Geometry: final body of the model. Coordinates: model frame, mm. A direction names the side the tool comes from. Give positions to 0.01 mm unless a question says otherwise; leave off trailing zeros. Write each loop counter-clockwise with the first axis right and the second up, starting at its lowest first coordinate (ties: lowest second). Pieces come first, ordered by that corner, then holes.
Autodesk Inventor part; units mm, degrees
ref_plane "YZ Plane" through (0, 0, 0) normal (1, 0, 0) x (0, 1, 0)
ref_plane "XZ Plane" through (0, 0, 0) normal (0, 1, 0) x (-1, 0, 0)
ref_plane "XY Plane" through (0, 0, 0) normal (0, 0, 1) x (1, 0, 0)
sketch "Sketch1" plane through (0, 0, 0) normal (0, 1, 0) x (-1, 0, 0)
  line L0 (0, 0) -> (25.4, 0)
  line L1 (25.4, 0) -> (25.4, -19.05)
  line L2 (25.4, -19.05) -> (0, -19.05)
  line L3 (0, -19.05) -> (0, 0)
  line L4 (25.4, -9.525) -> (38.1, -9.525)
  line L5 (38.1, -9.525) -> (34.3696, 9.525)
  line L6 (34.3696, 9.525) -> (0, 0)
  line L7 (38.1, -9.525) -> (34.3696, -28.575)
  line L8 (34.3696, -28.575) -> (0, -19.05)
  line L9 (-0.8514, -15.5194) -> (31.9128, -24.5995)
  line L10 (31.9128, -24.5995) -> (34.3908, -11.9449)
  line L11 (1.5358, -2.8691) -> (31.9128, 5.5495)
  line L12 (31.9128, 5.5495) -> (34.3903, -7.1024)
  line L13 (3.175, -19.05) -> (3.175, -6.35)
  line L14 (34.3908, -11.9449) -> (38.1, 8.3994)
  line L15 (34.3903, -7.1024) -> (39.9584, -35.5367)
  line L16 (3.175, -6.35) -> (3.175, -2.4148)
  point P0 (3.175, -19.05)
  point P1 (3.175, 0)
  point P2 (11.8883, 0)
  point P3 (34.7909, -6.35)
  point P4 (11.8883, -19.05)
  point P5 (3.175, -16.6352)
  point P6 (3.175, -2.6421)
  point P7 (0, -15.7553)
  point P8 (34.8478, -9.4386)
  dimension "d0" = 25.4
  dimension "d1" = 19.05
  dimension "d2" = 12.7
  dimension "d3" = 19.05
  dimension "d4" = 3.175
  dimension "d5" = 3.175
  dimension "d6" = 3.175
extrude "Extrusion1" add sketch "Sketch1" against normal blind 9.525 contours L6 L5 L14 L15 L12 L11 L0 | L0 L11 L16 L13 L9 L3 | L9 L13 L2 L3 | L2 L9 L10 L14 L4 L15 L7 L8 | L9 L2 L13 | L5 L4 L15 L14 | L7 L15 L4 | L15 L4 L14
sketch "Sketch3" plane through (-38.1, -9.525, -9.525) normal (-0.9814, 0, 0.1922) x (0.1922, 0, 0.9814)
  line L0 (0, 9.525) -> (19.4118, 9.525)
  circle A0 centre (9.7059, 9.525) radius 4.572
  point P0 (16.6692, 9.525)
  point P1 (14.2779, 9.525)
  point P2 (5.1339, 9.525)
  dimension "d12" = 9.144
extrude "Extrusion3" cut sketch "Sketch3" against normal blind 25.4 contours L0 A0 picked at (10.7462, 7.5625)
sketch "Sketch4" plane through (-34.3696, -9.525, -28.575) normal (-0.9814, 0, -0.1922) x (-0.1922, 0, 0.9814)
  line L0 (0, 9.525) -> (19.4118, 9.525)
  circle A0 centre (9.7059, 9.525) radius 4.572
  point P0 (21.4375, 9.525)
  point P1 (14.2779, 9.525)
  point P2 (5.1339, 9.525)
  dimension "d15" = 9.144
extrude "Extrusion4" cut sketch "Sketch4" against normal blind 25.4 contours L0 A0 picked at (10.7462, 7.5625)
sketch "Sketch5" plane through (-3.175, 0, -16.6352) normal (-1, 0, 0) x (0, 0, 1)
  line L0 (7.1966, 0) -> (4.6903, 0)
  circle A0 centre (7.1966, 0) radius 4.572
  point P0 (16.6352, 0)
  dimension "d18" = 9.144
extrude "Extrusion5" cut sketch "Sketch5" against normal blind 9.525
sketch "Sketch6" plane through (0, -9.525, 0) normal (0, -1, 0) x (1, 0, 0)
  line L0 (-34.3696, -28.575) -> (0, -19.05)
  line L1 (0, -19.05) -> (0, 0)
  line L2 (0, 0) -> (-34.3696, 9.525)
  line L3 (-34.3696, 9.525) -> (-38.1, -9.525)
  line L4 (-38.1, -9.525) -> (-34.3696, -28.575)
  line L5 (-3.175, -2.4148) -> (-3.175, -16.6352)
  line L6 (-3.175, -16.6352) -> (-31.9128, -24.5995)
  line L7 (-31.9128, -24.5995) -> (-34.3908, -11.9449)
  line L8 (-34.3908, -11.9449) -> (-34.8478, -9.4386)
  line L9 (-34.8478, -9.4386) -> (-31.9128, 5.5495)
  line L10 (-31.9128, 5.5495) -> (-3.175, -2.4148)
extrude "Extrusion6" add sketch "Sketch6" against normal blind 3.175 contours L4 L3 L2 L1 L0 | L5 L6 L7 L8 L9 L10
sketch "Sketch7" plane through (0, 0, 0) normal (0, 1, 0) x (1, 0, 0)
  line L0 (-34.3696, -9.525) -> (0, 0)
  circle A0 centre (-17.1848, -4.7625) radius 3.175
  line L1 (-10.5511, 0.3706) -> (-31.9128, -5.5495)
  line L2 (-34.3696, 28.575) -> (0, 19.05)
  circle A1 centre (-17.1848, 23.8125) radius 3.175
  line L3 (-31.9128, 24.5995) -> (-10.5511, 18.6794)
  point P0 (-20.2445, 24.6604)
  point P1 (-14.1251, 22.9646)
  point P2 (-14.1251, -3.9146)
  point P3 (-20.2445, -5.6104)
extrude "Extrusion7" add sketch "Sketch7" against normal blind 9.525 contours L0 A0 | A1 L2 picked at (-16.7975, -6.2491) picked at (-16.3793, 25.0421)
sketch "Sketch8" plane through (0, 0, 0) normal (0, 1, 0) x (1, 0, 0)
  arc A0 (-14.1251, 22.9646) -> (-20.2445, 24.6604) centre (-17.1848, 23.8125) ccw
  circle A1 centre (-17.1848, 23.8125) radius 1.5
  arc A2 (-20.2445, -5.6104) -> (-14.1251, -3.9146) centre (-17.1848, -4.7625) ccw
  circle A3 centre (-17.1848, -4.7625) radius 1.5
  point P0 (0, 0)
  dimension "d25" = 3
  dimension "d26" = 3
extrude "Extrusion8" cut sketch "Sketch8" against normal blind 9.525
sketch "Sketch10" plane through (-34.3696, -9.525, 9.525) normal (0.2671, 0, 0.9637) x (0.9637, 0, -0.2671)
  line L0 (25.5962, 9.525) -> (3.4293, 9.525)
  circle A0 centre (10.7027, 9.525) radius 1.778
  circle A1 centre (24.8175, 9.525) radius 1.778
  line L1 (21.0075, 9.525) -> (21.0075, 0)
  point P0 (35.665, 9.525)
  point P1 (14.5127, 9.525)
  point P2 (8.9247, 9.525)
  point P3 (12.4807, 9.525)
  dimension "d29" = 3.556
  dimension "d30" = 3.556
  dimension "d31" = 3.81
  dimension "d32" = 3.81
extrude "Extrusion9" cut sketch "Sketch10" against normal blind 9.525 contours A0 L0 | A1 picked at (11.0394, 9.0372)
properties part number "powerFromBatterySplitHousing"
Item 1: Section D-D, the plane x = -7. Return the cut outline in (y, z) (3 decimals), plus the area to 3 significant figures.
Found:
outline: (-9.525, -20.99) - (0, -20.99) - (0, -17.695) - (-6.35, -17.695) - (-6.35, -1.355) - (0, -1.355) - (0, 1.94) - (-9.525, 1.94) - close
area: 115 mm2
Item 2: Section C-C, the plane x = -31. Return the cut outline in (y, z) (3 decimals), plus the area to 3 significant figures.
Found:
outline: (-9.525, -27.641) - (0, -27.641) - (0, -24.347) - (-6.35, -24.347) - (-6.35, 5.297) - (0, 5.297) - (0, 8.591) - (-9.525, 8.591) - close
area: 157 mm2
Item 3: Pin query (flat end, axial travel): pin 1 Ø1.5 at (y, z) = (-5, -22) entering from -X; pin 2 Ø1.5 at (y, z) = (-1.5, -12.5) entering from +X; pin 3 Ø4 at (x, z) = (-24, -6) entering from +Y. Return the tip coordinate at first contact, or that it passes through.
Found:
pin 1: stops at x = -35.8
pin 2: stops at x = -34.14
pin 3: stops at y = -6.35
Item 4: Reachability of faces 5 (the face through (-17.3, -3.1, 1.5)), 6 (the face through (-18.683, -4.696, 4.697)) from +Z, -Z, +X, -X, +Y, -Y: full face, straight path, thin tool, end or side. Return the list, or none.
Found:
face 5: +Y
face 6: +Y, -Y
Item 5: Section A-A, the plane y = -2.5. State how many separate pieces and enclosed holes the cut face has, plus the area to 3 significant figures.
Found:
separate pieces: 3
enclosed holes: 2
area: 316 mm2
Item 6: Pull-direction query (X, two-part tool) for faces 1 (the face through (-33.134, -5.247, -18.361)), 2 (the face through (-24.511, -1.778, 5.169)), 3 (the face through (0, -6, -10)), 4 (the face through (-1.61, -4.57, -9.54)); classes: +X half, -X half, draft (parallel to the pull), parting line (faces both ways), or undercut.
Found:
face 1: undercut
face 2: undercut
face 3: +X half
face 4: draft
Item 7: Line query: L1, parallel to Z at x = -16, y = -3.25; L2, parallel to Z at x = -16.5, y = -2.75; L3, parallel to Y at x = -8, z = -17.5 (3 decimals). Output: solid intervals per line, ascending.
Found:
L1: z = -26.76 to -24.73, -22.89 to -20.19, 1.14 to 3.84, 5.68 to 7.71
L2: z = -26.91 to -25.15, -22.48 to -20.33, 1.28 to 3.43, 6.1 to 7.86
L3: y = -9.525 to -6.35
